from build123d import *

# Parameters (mm, degrees)
F1_DEPTH = 3


# Not quite as in the source:
# - a feature names something its author has since deleted; it is built from what else it names


with BuildPart() as f1:
    # F0 (on Top) → F1 (new body)
    with BuildSketch(Plane.XY):
        with BuildLine():
            ThreePointArc((0.6180339887, 25.7372071924), (0, 25.639320225), (-0.6180339887, 25.7372071924))
            Line((-0.6180339887, 25.7372071924), (-6.2054140173, 8.5410196625))
            Line((-6.2054140173, 8.5410196625), (-26.286555606, 8.5410196625))
            Line((-26.286555606, 8.5410196625), (-10.0405707943, -3.2623792125))
            Line((-10.0405707943, -3.2623792125), (-16.2459848116, -22.360679775))
            Line((-16.2459848116, -22.360679775), (0, -10.5572809))
            Line((0, -10.5572809), (16.2459848116, -22.360679775))
            Line((16.2459848116, -22.360679775), (10.0405707943, -3.2623792125))
            Line((10.0405707943, -3.2623792125), (26.286555606, 8.5410196625))
            Line((26.286555606, 8.5410196625), (6.2054140173, 8.5410196625))
            Line((6.2054140173, 8.5410196625), (0.6180339887, 25.7372071924))
        make_face()
        with BuildLine():
            ThreePointArc((0.3090169944, 26.6882637087), (0, 26.639320225), (-0.3090169944, 26.6882637087))
            Line((-0.3090169944, 26.6882637087), (-0.6180339887, 25.7372071924))
            ThreePointArc((-0.6180339887, 25.7372071924), (0, 25.639320225), (0.6180339887, 25.7372071924))
            Line((0.6180339887, 25.7372071924), (0.3090169944, 26.6882637087))
        make_face()
        with BuildLine():
            Line((1.6180339887, 26.4637497204), (0.8090169944, 27.0515349727))
            ThreePointArc((0.8090169944, 27.0515349727), (0.5877852523, 26.8303032306), (0.3090169944, 26.6882637087))
            Line((0.3090169944, 26.6882637087), (0.6180339887, 25.7372071924))
            ThreePointArc((0.6180339887, 25.7372071924), (1.1755705046, 26.0212862363), (1.6180339887, 26.4637497204))
        make_face()
        with BuildLine():
            ThreePointArc((1, 27.639320225), (0.9510565163, 27.3303032306), (0.8090169944, 27.0515349727))
            Line((0.8090169944, 27.0515349727), (1.6180339887, 26.4637497204))
            ThreePointArc((1.6180339887, 26.4637497204), (1.9021130326, 27.0212862363), (2, 27.639320225))
            ThreePointArc((2, 27.639320225), (-0.6180339887, 29.5414332576), (-1.6180339887, 26.4637497204))
            Line((-1.6180339887, 26.4637497204), (-0.8090169944, 27.0515349727))
            ThreePointArc((-0.8090169944, 27.0515349727), (-0.3090169944, 28.5903767413), (1, 27.639320225))
        make_face()
        with BuildLine():
            ThreePointArc((-0.3090169944, 26.6882637087), (-0.5877852523, 26.8303032306), (-0.8090169944, 27.0515349727))
            Line((-0.8090169944, 27.0515349727), (-1.6180339887, 26.4637497204))
            ThreePointArc((-1.6180339887, 26.4637497204), (-1.1755705046, 26.0212862363), (-0.6180339887, 25.7372071924))
            Line((-0.6180339887, 25.7372071924), (-0.3090169944, 26.6882637087))
        make_face()
    extrude(amount=F1_DEPTH)


solid = f1.part
Check sheet for the modelled part. Datum: model origin and axes. Units: mm. A direction names the side the tool comes from. Coordinates: 2 decimals unless noted, no trailing zeros. Write each loop counter-clockwise with the first axis right and the second up, starting at its lowest first coordinate (ties: lowest second). Pieces come first, ordered by that corner, then holes.
Item 1: Cross-section at A-A on z = 1.2. Record the boundary of the cut face in (x, y).
Numbers:
outline: (-26.29, 8.54) - (-10.04, -3.26) - (-16.25, -22.36) - (0, -10.56) - (16.25, -22.36) - (10.04, -3.26) - (26.29, 8.54) - (6.21, 8.54) - (0.62, 25.74) arc R2 ccw (long way) to (-0.62, 25.74) - (-6.21, 8.54) - close; hole circle Ø2 at (0, 27.64)
Item 2: Depth check by flat-ended pin: pin 1 Ø12 at (x, y) = (14, -9) entering from +Z; pin 2 Ø1.5 at (x, z) = (-11.5, 2) entering from +Y; pin 3 Ø8 at (x, y) = (-8, 17.5) entering from -Z. Enter the tip coordinate at first touch or a pass-through.
Numbers:
pin 1: stops at z = 3
pin 2: stops at y = 8.54
pin 3: passes through
Item 3: Cross-section at B-B on x = 11.5. Record the boundary of the cut face in (y, z).
Numbers:
outline: (-18.91, 0) - (-7.75, 0) - (-7.75, 3) - (-18.91, 3) - close; (-2.2, 0) - (8.54, 0) - (8.54, 3) - (-2.2, 3) - close
Item 4: Mould release check, pull along Y, two halves, no side actions. Record for faces 1 (the face through (16, 8.541, 1)), 2 (the face through (-8.237, -16.542, 1.479)), 3 (the face through (18.05, 2.557, 1.479)): released by +Y, released by -Y, zero draft, split by the parting line, or undercut.
Numbers:
face 1: released by +Y
face 2: released by -Y
face 3: undercut
Item 5: Cross-section at D-D on x = -3.5. Record the boundary of the cut face in (y, z).
Numbers:
outline: (-13.1, 0) - (16.87, 0) - (16.87, 3) - (-13.1, 3) - close
Item 6: Access from +Z, -Z, +X, -X, +Y, -Y to the whole of each face (thin tool, end or side, straight path). Record for faces 4 (the face through (8.009, -16.376, 1.479)), 5 (the face through (3.45, 17.02, 1.48)), 6 (the face through (0, 0, 0)), 7 (the face through (-16, 8.541, 1)), 8 (the face through (-18.277, 2.722, 1.479)).
Numbers:
face 4: +Z, -Z, -Y
face 5: +Z, -Z, +X
face 6: -Z, +X, -X, +Y, -Y
face 7: +Z, -Z, -X, +Y
face 8: +Z, -Z, -X
Item 7: Scan lines: probe 1 along Y at (x, z) = (0, 1.8); probe 2 along X at (y, z) = (-14.5, 1.9); probe 3 along X at (y, z) = (-19.5, 0.35). Record each from-to range of solid material in increasing order.
Numbers:
probe 1: y = -10.56 to 26.64, 28.64 to 29.64
probe 2: x = -13.69 to -5.43, 5.43 to 13.69
probe 3: x = -15.32 to -12.31, 12.31 to 15.32
Item 8: Cross-section at C-C on y = -18. Record the boundary of the cut face in (x, z), then the cut area to 3 significant figures.
Numbers:
outline: (-14.83, 0) - (-10.24, 0) - (-10.24, 3) - (-14.83, 3) - close; (10.24, 0) - (14.83, 0) - (14.83, 3) - (10.24, 3) - close
area: 27.5 mm2
